Design review of the part built by this model. Coordinates are the model's own, in mm. Give positions to 0.01 mm unless a question says otherwise; leave off trailing zeros. Loops run counter-clockwise (first coordinate to the right, second up) from the corner with the lowest first, then second, coordinate; pieces in that order, holes last. Notation, with made-up numbers: (-22, -10) -> (15, -10) arc R13 ccw to (15, 12) -> close; hole circle Ø7 at (-1.75, -24). An arc over 180 degrees is marked (long way). Use a Markdown table: item, result. Add a question column.
1. Add section A-A (y = 419). State the section outline as (x, z) points, and give its area (3 significant figures).
2. For pin 1 Ø10 at (y, z) = (200, -17.5) entering from -X; pin 2 Ø8 at (y, z) = (128.5, -30) entering from -X; pin 3 Ø12 at (y, z) = (82, -11) entering from -X, all flat-tipped, find the tip position at first contact; note any pin that passes through.
3. Draft analysis for pull direction X (two halves, no side actions). For faces 1 (the flat face through (114.95, 128.88, -10.89)), 2 (the flat face through (131.895, 111.301, -17.902)), 3 (the cylindrical face through (260.8, 460.1, -0.1)), state which applies: pulls with the +X half, pulls with the -X half, needs draft (parallel to the pull), parting line crosses it, or undercut.
4. Add section B-B (x = 196). State the section outline as (y, z) points.
```python
from build123d import *

# Parameters (mm, degrees)
SKETCH2_R           = 12.7
SKETCH2_R_2         = 3.2639
SKETCH2_R_3         = 4.19989
BOSS_EXTRUDE1_DEPTH = 3.175


with BuildPart() as part:
    # Sketch2 → Boss-Extrude1 (new, symmetric)
    # profile 1 of 7: a face of its own
    with BuildSketch(Plane(origin=(0, 0, 0), x_dir=(0.9683571483215458, 0.03640581426885692, -0.2468988658985399), z_dir=(0.24956849419460725, -0.14125913850417393, 0.9579986547456604))):
        with BuildLine():
            Line((242.448329145, 239.243930423), (-8.577063088, 9.366108518))
            ThreePointArc((-8.577063088, 9.366108518), (5.11670298, 11.623654787), (12.7, 0))
            ThreePointArc((12.7, 0), (11.623654787, -5.11670298), (8.577063088, -9.366108518))
            Line((8.577063088, -9.366108518), (267.433066466, 227.682636686))
            ThreePointArc((267.433066466, 227.682636686), (253.522604962, 225.522910686), (246.164904285, 237.524143805))
            Line((246.164904285, 237.524143805), (246.363634717, 242.829392073))
            Line((246.363634717, 242.829392073), (242.448329145, 239.243930423))
        make_face()
    # profile 2 of 7: a face of its own
    with BuildSketch(Plane(origin=(0, 0, 0), x_dir=(0.9683571483215458, 0.03640581426885692, -0.2468988658985399), z_dir=(0.24956849419460725, -0.14125913850417393, 0.9579986547456604))):
        Circle(SKETCH2_R)
        with Locations(Location((0, 0, 0), (0, 0, 357.892497398))):
            Circle(SKETCH2_R_2, mode=Mode.SUBTRACT)
    # profile 3 of 7: a face of its own
    with BuildSketch(Plane(origin=(0, 0, 0), x_dir=(0.9683571483215458, 0.03640581426885692, -0.2468988658985399), z_dir=(0.24956849419460725, -0.14125913850417393, 0.9579986547456604))):
        with Locations((258.856003378, 237.048745204)):
            Circle(SKETCH2_R)
        with Locations(Location((258.856003378, 237.048745204, 0), (0, 0, 357.892497398))):
            Circle(SKETCH2_R_2, mode=Mode.SUBTRACT)
    # profile 4 of 7: a face of its own
    with BuildSketch(Plane(origin=(0, 0, 0), x_dir=(0.9683571483215458, 0.03640581426885692, -0.2468988658985399), z_dir=(0.24956849419460725, -0.14125913850417393, 0.9579986547456604))):
        with BuildLine():
            Line((246.562365149, 248.134640341), (246.363634717, 242.829392073))
            Line((246.363634717, 242.829392073), (250.278940289, 246.414853723))
            ThreePointArc((250.278940289, 246.414853723), (263.972706358, 248.672399992), (271.556003378, 237.048745204))
            ThreePointArc((271.556003378, 237.048745204), (271.553777956, 236.811004245), (271.54710247, 236.573346604))
            Line((271.54710247, 236.573346604), (279.589066496, 451.259216922))
            ThreePointArc((279.589066496, 451.259216922), (266.422568803, 439.04351643), (254.206868311, 452.210014123))
            Line((254.206868311, 452.210014123), (246.562365149, 248.134640341))
        make_face()
    # profile 5 of 7: a face of its own
    with BuildSketch(Plane(origin=(0, 0, 0), x_dir=(0.9683571483215458, 0.03640581426885692, -0.2468988658985399), z_dir=(0.24956849419460725, -0.14125913850417393, 0.9579986547456604))):
        with BuildLine():
            Line((250.278940289, 246.414853723), (246.363634717, 242.829392073))
            Line((246.363634717, 242.829392073), (246.164904285, 237.524143805))
            ThreePointArc((246.164904285, 237.524143805), (247.330168859, 242.38214362), (250.278940289, 246.414853723))
        make_face()
    # profile 6 of 7: a face of its own
    with BuildSketch(Plane(origin=(0, 0, 0), x_dir=(0.9683571483215458, 0.03640581426885692, -0.2468988658985399), z_dir=(0.24956849419460725, -0.14125913850417393, 0.9579986547456604))):
        with Locations((266.897967404, 451.734615523)):
            Circle(SKETCH2_R)
        with Locations(Location((266.897967404, 451.734615523, 0), (0, 0, 357.892497398))):
            Circle(SKETCH2_R_3, mode=Mode.SUBTRACT)
    # profile 7 of 7: a face of its own
    with BuildSketch(Plane(origin=(0, 0, 0), x_dir=(0.9683571483215458, 0.03640581426885692, -0.2468988658985399), z_dir=(0.24956849419460725, -0.14125913850417393, 0.9579986547456604))):
        with BuildLine():
            ThreePointArc((246.562365149, 248.134640341), (245.397100575, 243.276640526), (242.448329145, 239.243930423))
            Line((242.448329145, 239.243930423), (246.363634717, 242.829392073))
            Line((246.363634717, 242.829392073), (246.562365149, 248.134640341))
        make_face()
    extrude(amount=BOSS_EXTRUDE1_DEPTH, both=True)


solid = part.part
```
Taken from the geometry:
| question | item | result |
|---|---|---|
| 1 | outline | (243.98, -5.09) -> (268.56, -11.49) -> (270.17, -5.29) -> (245.59, 1.12) -> close |
| 1 | area | 163 mm^2 |
| 2 | pin 1 | stops at x = 183.06 |
| 2 | pin 2 | passes through |
| 2 | pin 3 | stops at x = 60.36 |
| 3 | face 1 | pulls with the -X half |
| 3 | face 2 | pulls with the +X half |
| 3 | face 3 | undercut |
| 4 | outline | (172.48, -22.31) -> (174.92, -28.58) -> (209, -23.56) -> (206.56, -17.29) -> close |
